The model under review builds one solid part; all positions refer to its coordinate system, in mm. Coordinates: 2 decimals unless noted, no trailing zeros. Order: outer loops, then holes, each group sorted by start corner. A loop starts at its lowest first (then second) coordinate and runs counter-clockwise, first axis right, second up. Notation, with made-up numbers: (35, 1) - (65, 1) arc R28 ccw to (65, 31) - close; hole circle Ø5 at (16, 28.5). An arc over 180 degrees is marked (long way). Answer in a Markdown table with one row per item.
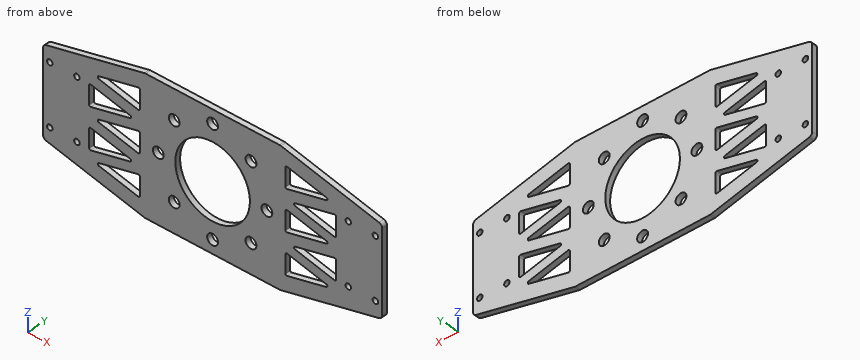
```python
from build123d import *

# Parameters (mm, degrees)
SKETCH_1_R          = 2.05
SKETCH_1_R_2        = 4
EXTRUDE_1_DEPTH     = 4
SKETCH_5_R          = 27.5
CUT_EXTRUDE_5_DEPTH = 10
FILLET_2_R          = 3
FILLET_3_R          = 5
CUT_EXTRUDE_6_DEPTH = 10
FILLET_4_R          = 1


with BuildPart() as part:
    # 草图1 → 凸台-拉伸1 (new body)
    with BuildSketch(Plane(origin=(0, 0, 0), x_dir=(1, 0, 0), z_dir=(0, 1, 0))):
        Polygon((-49.840999723, 50), (-125, 32.5), (-125, -32.5), (-49.840999723, -50), (49.840999723, -50), (125, -32.5), (125, 32.5), (49.840999723, 50), align=None)
        with Locations(Location((-120, -22.5, 0), (0, 0, 270))):
            Circle(SKETCH_1_R, mode=Mode.SUBTRACT)
        with Locations(Location((-100, -22.5, 0), (0, 0, 270))):
            Circle(SKETCH_1_R, mode=Mode.SUBTRACT)
        with Locations(Location((-120, 22.5, 0), (0, 0, 270))):
            Circle(SKETCH_1_R, mode=Mode.SUBTRACT)
        with Locations(Location((-100, 22.5, 0), (0, 0, 270))):
            Circle(SKETCH_1_R, mode=Mode.SUBTRACT)
        with Locations(Location((0, 40, 0), (0, 0, 270))):
            Circle(SKETCH_1_R_2, mode=Mode.SUBTRACT)
        with Locations(Location((-28.284271247, -28.284271247, 0), (0, 0, 270))):
            Circle(SKETCH_1_R_2, mode=Mode.SUBTRACT)
        with Locations(Location((-40, 0, 0), (0, 0, 270))):
            Circle(SKETCH_1_R_2, mode=Mode.SUBTRACT)
        with Locations(Location((0, -40, 0), (0, 0, 270))):
            Circle(SKETCH_1_R_2, mode=Mode.SUBTRACT)
        with Locations(Location((28.284271247, -28.284271247, 0), (0, 0, 270))):
            Circle(SKETCH_1_R_2, mode=Mode.SUBTRACT)
        with Locations(Location((-28.284271247, 28.284271247, 0), (0, 0, 270))):
            Circle(SKETCH_1_R_2, mode=Mode.SUBTRACT)
        with Locations(Location((40, 0, 0), (0, 0, 270))):
            Circle(SKETCH_1_R_2, mode=Mode.SUBTRACT)
        with Locations(Location((28.284271247, 28.284271247, 0), (0, 0, 270))):
            Circle(SKETCH_1_R_2, mode=Mode.SUBTRACT)
        with Locations(Location((120, 22.5, 0), (0, 0, 270))):
            Circle(SKETCH_1_R, mode=Mode.SUBTRACT)
        with Locations(Location((100, 22.5, 0), (0, 0, 270))):
            Circle(SKETCH_1_R, mode=Mode.SUBTRACT)
        with Locations(Location((100, -22.5, 0), (0, 0, 270))):
            Circle(SKETCH_1_R, mode=Mode.SUBTRACT)
        with Locations(Location((120, -22.5, 0), (0, 0, 270))):
            Circle(SKETCH_1_R, mode=Mode.SUBTRACT)
    extrude(amount=EXTRUDE_1_DEPTH)

    # 草图5 → 切除-拉伸5 (cut)
    with BuildSketch(Plane(origin=(0, 4, 0), x_dir=(1, 0, 0), z_dir=(0, 1, 0))):
        with Locations(Location((0, 0, 0), (0, 0, 270))):
            Circle(SKETCH_5_R)
    extrude(amount=-CUT_EXTRUDE_5_DEPTH, mode=Mode.SUBTRACT)

    # 圆角2
    fillet_2_edges = [part.edges().sort_by_distance(p)[0] for p in [
        (-125, 2, 32.5),
        (-125, 2, -32.5),
        (125, 2, -32.5),
        (125, 2, 32.5),
    ]]
    fillet(fillet_2_edges, radius=FILLET_2_R)

    # 圆角3
    fillet_3_edges = [part.edges().sort_by_distance(p)[0] for p in [
        (-49.840999723, 2, 50),
        (-49.840999723, 2, -50),
        (49.840999723, 2, -50),
        (49.840999723, 2, 50),
    ]]
    fillet(fillet_3_edges, radius=FILLET_3_R)

    # 草图6 → 切除-拉伸6 (cut)
    with BuildSketch(Plane(origin=(0, 4, 0), x_dir=(1, 0, 0), z_dir=(0, 1, 0))):
        Polygon((-88, 30), (-53.641599874, 38), (-53.641599874, 22), align=None)
        Polygon((-53.641599874, -8), (-88, 0), (-53.641599874, 8), align=None)
        Polygon((-53.641599874, -38), (-88, -30), (-53.641599874, -22), align=None)
        Polygon((-91, 23.511273333), (-91, 7.511273333), (-56.641599874, 15.511273333), align=None)
        Polygon((-56.641599874, -14.488726667), (-91, -6.488726667), (-91, -22.488726667), align=None)
        Polygon((53.641599874, -22), (53.641599874, -38), (88, -30), align=None)
        Polygon((91, -22.488726667), (56.641599874, -14.488726667), (91, -6.488726667), align=None)
        Polygon((91, 7.511273333), (56.641599874, 15.511273333), (91, 23.511273333), align=None)
        Polygon((53.641599874, 8), (53.641599874, -8), (88, 0), align=None)
        Polygon((53.641599874, 38), (53.641599874, 22), (88, 30), align=None)
    extrude(amount=-CUT_EXTRUDE_6_DEPTH, mode=Mode.SUBTRACT)

    # 圆角4
    fillet_4_edges = [part.edges().sort_by_distance(p)[0] for p in [
        (-88, 2, 30),
        (-53.641599874, 2, 22),
        (-53.641599874, 2, 38),
        (-91, 2, 22.488726667),
        (-91, 2, 6.488726667),
        (-56.641599874, 2, 14.488726667),
        (-91, 2, -23.511273333),
        (-56.641599874, 2, -15.511273333),
        (-91, 2, -7.511273333),
        (-88, 2, 0),
        (-53.641599874, 2, -8),
        (-53.641599874, 2, 8),
        (91, 2, -23.511273333),
        (91, 2, -7.511273333),
        (56.641599874, 2, -15.511273333),
        (53.641599874, 2, -8),
        (88, 2, 0),
        (53.641599874, 2, 8),
        (53.641599874, 2, 22),
        (88, 2, 30),
        (53.641599874, 2, 38),
        (91, 2, 6.488726667),
        (91, 2, 22.488726667),
        (56.641599874, 2, 14.488726667),
        (53.641599874, 2, -38),
        (88, 2, -30),
        (53.641599874, 2, -22),
        (-53.641599874, 2, -22),
        (-88, 2, -30),
        (-53.641599874, 2, -38),
    ]]
    fillet(fillet_4_edges, radius=FILLET_4_R)


solid = part.part
```
Item 1: We need section D-D, the plane y = 1.7. State how many separate pieces and enclosed holes the cut face has, then the cut area to 3 significant figures.
Check values:
| item | result |
|---|---|
| separate pieces | 1 |
| enclosed holes | 27 |
| area | 16,800 mm^2 |
Item 2: We need section A-A, the plane x = -40. Write out the cut boundary in (y, z).
Check values:
| item | result |
|---|---|
| outline | (0, -50) - (4, -50) - (4, -4) - (0, -4) - close; (0, 4) - (4, 4) - (4, 50) - (0, 50) - close |
Item 3: Clearance check with a flat-ended pin moving along its axis: pin 1 Ø1.5 at (y, z) = (3, -33) entering from -X. State where the tip first meets the part, or that it passes through.
Check values:
| item | result |
|---|---|
| pin 1 | x = -124.11 |
Item 4: We need section B-B, the plane z = -40. Write out the cut boundary in (x, y).
Check values:
| item | result |
|---|---|
| outline | (-92.79, 0) - (-4, 0) - (-4, 4) - (-92.79, 4) - close; (4, 0) - (92.79, 0) - (92.79, 4) - (4, 4) - close |
Item 5: We need section C-C, the plane x = 87.5. Write out the cut boundary in (y, z).
Check values:
| item | result |
|---|---|
| outline | (0, -41.23) - (4, -41.23) - (4, -22.7) - (0, -22.7) - close; (0, -8.33) - (4, -8.33) - (4, 7.3) - (0, 7.3) - close; (0, 21.67) - (4, 21.67) - (4, 41.23) - (0, 41.23) - close |
Item 6: To check wall thickness, follow line 1 (Z direction, x = 99, y = 2.05); line 2 (Z direction, x = 29, y = 0.9); line 3 (Z direction, x = -78, y = 0.5). State the ranges of each line that lie inside material, in increasing order. Write a range as from..to.
Check values:
| item | result |
|---|---|
| line 1 | -38.55..-24.29, -20.71..20.71, 24.29..38.55 |
| line 2 | -50..-32.22, -24.35..24.35, 32.22..50 |
| line 3 | -43.44..-32.33, -27.67..-20.48, -10.54..-2.33, 2.33..9.52, 19.46..27.67, 32.33..43.44 |
